Geometry check sheet. Reference: the model listing, model coordinates, mm. Coordinates: 2 decimals unless noted, no trailing zeros. Order: outer loops, then holes, each group sorted by start corner. A loop starts at its lowest first (then second) coordinate and runs counter-clockwise, first axis right, second up. Notation, with made-up numbers: (1.5, -39) - (41.5, -39) arc R23 ccw to (41.5, -16) - close; hole circle Ø8 at (74.5, 32). An arc over 180 degrees is marked (long way). Return JSON: item names as keys, results as strings. Group by question number.
Item 1: Section check A-A on x = -2.5. Enter the section's corners in (y, z), then the cut area to 3 significant figures.
Item 2: Scan lines: probe 1 along Z at (x, y) = (-1.65, -117); probe 2 along Y at (x, z) = (-3.3, 42.5); probe 3 along Z at (x, y) = (-4, -43.5). Record each from-to range of solid material in increasing order.
Item 3: Section check B-B on z = 61.5. Enter the section's corners in (x, y), then the cut area to 4 significant figures.
Item 4: Section check C-C on y = -59. Enter the section's corners in (x, z), then the cut area to 3 significant figures.
Item 5: Gauge pin test, flat end, axial feed: pin 1 (2.5 mm diameter, centred on x = -2.5, z = 101, fed in from +Y). Record the tip position at first contact, or that the pin passes through.
Solid Edge part; units mm, degrees
sketch "Sketch1" plane through (0, 0, 0) normal (1, 0, 0) x (0, 1, 0)
  line L0 (-136.5657, 103.3324) -> (-126.5657, 103.3324)
  line L1 (-126.5657, 103.3324) -> (-126.5657, 96.3324)
  line L2 (-126.5657, 96.3324) -> (-106.5657, 96.3324)
  line L3 (-106.5657, 96.3324) -> (-106.5657, 103.3324)
  line L4 (-106.5657, 103.3324) -> (-14.0657, 103.3324)
  line L5 (-14.0657, 103.3324) -> (-14.0657, 96.3324)
  line L6 (-14.0657, 96.3324) -> (5.9343, 96.3324)
  line L7 (5.9343, 96.3324) -> (5.9343, 8.3324)
  line L8 (5.9343, 8.3324) -> (-41.5657, 8.3324)
  line L9 (-41.5657, 8.3324) -> (-41.5657, 13.3324)
  line L10 (-41.5657, 13.3324) -> (-89.0657, 13.3324)
  line L11 (-89.0657, 13.3324) -> (-89.0657, 8.3324)
  line L12 (-89.0657, 8.3324) -> (-136.5657, 8.3324)
  line L13 (-136.5657, 8.3324) -> (-136.5657, 28.3324)
  line L14 (-136.5657, 28.3324) -> (-131.5657, 28.3324)
  line L15 (-131.5657, 28.3324) -> (-131.5657, 78.3324)
  line L16 (-131.5657, 78.3324) -> (-136.5657, 78.3324)
  line L17 (-136.5657, 78.3324) -> (-136.5657, 103.3324)
  dimension "D1" = 126.5657
  dimension "D2" = 126.5657
  dimension "D3" = 136.5657
  dimension "D4" = 131.5657
  dimension "D5" = 136.5657
  dimension "D6" = 131.5657
extrude "Protrusion1" add sketch "Sketch1" against normal blind 5
properties material "Acier"
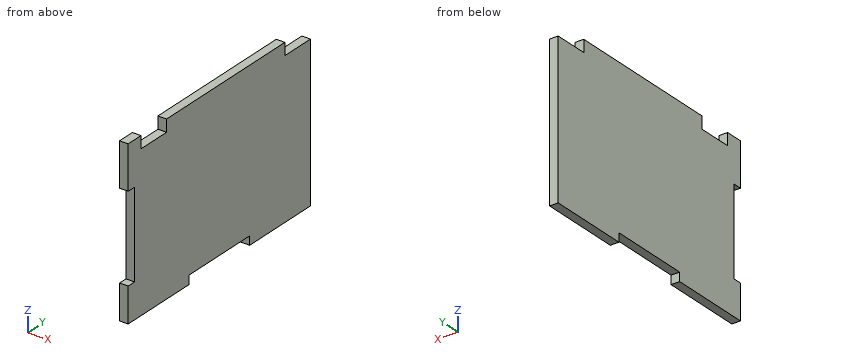
Computed:
{
 "1": {"outline": "(-136.57, 8.33) - (-89.07, 8.33) - (-89.07, 13.33) - (-41.57, 13.33) - (-41.57, 8.33) - (5.93, 8.33) - (5.93, 96.33) - (-14.07, 96.33) - (-14.07, 103.33) - (-106.57, 103.33) - (-106.57, 96.33) - (-126.57, 96.33) - (-126.57, 103.33) - (-136.57, 103.33) - (-136.57, 78.33) - (-131.57, 78.33) - (-131.57, 28.33) - (-136.57, 28.33) - close", "area": "12,800 mm²"},
 "2": {"probe 1": "z = 8.33 to 96.33", "probe 2": "y = -131.57 to 5.93", "probe 3": "z = 13.33 to 103.33"},
 "3": {"outline": "(-5, -131.57) - (0, -131.57) - (0, 5.93) - (-5, 5.93) - close", "area": "687.5 mm²"},
 "4": {"outline": "(-5, 13.33) - (0, 13.33) - (0, 103.33) - (-5, 103.33) - close", "area": "450 mm²"},
 "5": {"pin 1": "stops at y = -14.07"}
}
